Verification items for the finished model (mm, model axes). Round coordinates to 2 decimals unless told otherwise and drop trailing zeros. Write each loop counter-clockwise with the first axis right and the second up, starting at its lowest first coordinate (ties: lowest second). Pieces come first, ordered by that corner, then holes. Notation, with made-up numbers: (-32, -24) -> (9, -24) arc R11 cw to (9, -6) -> close; hole circle Ø9 at (63, 86.25). An arc over 180 degrees is marked (long way). Answer as a JSON object with one key per item and string values. Group by question number.
(1) Draft check along Y on faces 1 (the face through (33.81, 20.57, 2.46)), 2 (the face through (25, 7, 0)), 3 (the face through (-4.85, -1.21, 2.46)). Enter one of: released by +Y, released by -Y, zero draft, split by the parting line, or undercut.
(2) Sectioned sample at C-C on x = 30. Record the cut outline in (y, z).
(3) Sectioned sample at A-A on z = 1.75. Record the cut outline in (x, y).
(4) Scan lines: L1, parallel to Y at x = 28.5, z = 3.25; L2, parallel to Y at x = -1.5, z = 1.6; L3, parallel to X at y = -1, z = 4.85. Record each from-to range of solid material in increasing order. Write a range as from..to.
(5) Sectioned sample at D-D on y = 11. Record the cut outline in (x, z), and give its area (3 significant figures).
(6) Sectioned sample at B-B on y = 20.5. Record the cut outline in (x, z), and give its area (3 significant figures).
(7) Gauge pin test, flat ends, axial feed: pin 1 Ø4 at (x, y) = (18, 17.5) entering from +Z; pin 2 Ø3 at (y, z) = (10.5, 2.5) entering from +X; pin 3 Ø1.5 at (y, z) = (20.5, 4) entering from +X. Record the tip position at first contact, or that the pin passes through.
```python
from build123d import *

# Parameters (mm, degrees)
SKETCH_1_R      = 1.7
EXTRUDE_1_DEPTH = 5


with BuildPart() as part:
    # ｽｹｯﾁ1 → ﾎﾞｽ - 押し出し1 (new body)
    with BuildSketch(Plane.XY):
        with BuildLine():
            Line((54.082739258, 2.886388773), (39.5897808, 23.386388791))
            ThreePointArc((39.5897808, 23.386388791), (36.578191054, 25.383916333), (33.007041847, 24.830127187))
            Line((33.007041847, 24.830127187), (-2.50000007, 4.330126978))
            ThreePointArc((-2.50000007, 4.330126978), (-4.829629126, -1.294095246), (-3.8e-08, -5))
            Line((-3.8e-08, -5), (50, -5))
            ThreePointArc((50, -5), (54.440267102, -2.298701387), (54.082739258, 2.886388773))
        make_face()
        Circle(SKETCH_1_R, mode=Mode.SUBTRACT)
        with Locations((30, 0)):
            Circle(SKETCH_1_R, mode=Mode.SUBTRACT)
        with Locations((35.507041555, 20.5)):
            Circle(SKETCH_1_R, mode=Mode.SUBTRACT)
        with Locations((50, 0)):
            Circle(SKETCH_1_R, mode=Mode.SUBTRACT)
    extrude(amount=EXTRUDE_1_DEPTH)


solid = part.part
```
Computed values:
{
 "1": {"face 1": "undercut", "face 2": "zero draft", "face 3": "split by the parting line"},
 "2": {"outline": "(-5, 0) -> (-1.7, 0) -> (-1.7, 5) -> (-5, 5) -> close; (1.7, 0) -> (23.09, 0) -> (23.09, 5) -> (1.7, 5) -> close"},
 "3": {"outline": "(-2.5, 4.33) arc R5 ccw to (0, -5) -> (50, -5) arc R5 ccw to (54.08, 2.89) -> (39.59, 23.39) arc R5 ccw to (33.01, 24.83) -> close; hole circle Ø3.4 at (0, 0); hole circle Ø3.4 at (30, 0); hole circle Ø3.4 at (35.51, 20.5); hole circle Ø3.4 at (50, 0)"},
 "4": {"L1": "-5..-0.8, 0.8..22.23", "L2": "-4.77..-0.8, 0.8..4.91", "L3": "-4.9..-1.37, 1.37..28.63, 31.37..48.63, 51.37..54.9"},
 "5": {"outline": "(9.05, 0) -> (48.35, 0) -> (48.35, 5) -> (9.05, 5) -> close", "area": "196 mm2"},
 "6": {"outline": "(25.51, 0) -> (33.81, 0) -> (33.81, 5) -> (25.51, 5) -> close; (37.21, 0) -> (41.63, 0) -> (41.63, 5) -> (37.21, 5) -> close", "area": "63.6 mm2"},
 "7": {"pin 1": "z = 5", "pin 2": "x = 49.76", "pin 3": "x = 42.16"}
}
